The listing builds one solid part. Answer for the finished solid, in the listing's coordinates (mm). A direction names the side the tool comes from. Coordinates: 2 decimals unless noted, no trailing zeros. Order: outer loops, then holes, each group sorted by start corner. A loop starts at its lowest first (then second) coordinate and runs counter-clockwise, first axis right, second up. Notation, with made-up numbers: (49, 38.5) -> (94, 38.5) arc R17 cw to (94, 69.5) -> close; hole circle Ø1 at (75, -40). An arc over 180 degrees is marked (long way). Answer in a Markdown table with one row per item. Add a question column.
```python
from build123d import *

# Parameters (mm, degrees)
ESQUISSE1_W             = 200
ESQUISSE1_H             = 220
BOSS_EXTRU_1_DEPTH      = 15
ESQUISSE2_R             = 4
ENL_V_MAT_EXTRU_1_DEPTH = 6
ENL_V_MAT_EXTRU_2_DEPTH = 1.6
ENL_V_MAT_EXTRU_3_DEPTH = 5


with BuildPart() as part:
    # Esquisse1 → Boss.-Extru.1 (new body)
    with BuildSketch(Plane.XY):
        with Locations((100, 110)):
            Rectangle(ESQUISSE1_W, ESQUISSE1_H)
    extrude(amount=BOSS_EXTRU_1_DEPTH)

    # Esquisse2 → Enlèv. mat.-Extru.1 (cut)
    with BuildSketch(Plane.XY.offset(15)):
        with Locations((74.322, 91.45)):
            Circle(ESQUISSE2_R)
        with Locations((74.322, 153.45)):
            Circle(ESQUISSE2_R)
        with Locations((114.822, 91.45)):
            Circle(ESQUISSE2_R)
        with Locations((114.822, 153.45)):
            Circle(ESQUISSE2_R)
    extrude(amount=-ENL_V_MAT_EXTRU_1_DEPTH, mode=Mode.SUBTRACT)

    # Esquisse3 → Enlèv. mat.-Extru.2 (cut)
    with BuildSketch(Plane.XY.offset(15)):
        Polygon((27, 50), (27, 24.928776057), (74, 24.928776057), (74, 49.915697098), (124.85, 49.915697098), (124.85, 189.875697098), (25, 189.875697098), (25, 50), align=None)
    extrude(amount=-ENL_V_MAT_EXTRU_2_DEPTH, mode=Mode.SUBTRACT)

    # Esquisse4 → Enlèv. mat.-Extru.3 (cut)
    with BuildSketch(Plane.XY.offset(15)):
        with BuildLine():
            Line((106.85, 182.875697098), (101.85, 182.875697098))
            ThreePointArc((101.85, 182.875697098), (98.314466094, 181.411231003), (96.85, 177.875697098))
            Line((96.85, 177.875697098), (96.85, 65.875697098))
            ThreePointArc((96.85, 65.875697098), (98.314466094, 62.340163192), (101.85, 60.875697098))
            Line((101.85, 60.875697098), (106.85, 60.875697098))
            ThreePointArc((106.85, 60.875697098), (110.385533906, 62.340163192), (111.85, 65.875697098))
            Line((111.85, 65.875697098), (111.85, 177.875697098))
            ThreePointArc((111.85, 177.875697098), (110.385533906, 181.411231003), (106.85, 182.875697098))
        make_face()
        with BuildLine():
            Line((87.85, 60.875697098), (82.85, 60.875697098))
            ThreePointArc((82.85, 60.875697098), (79.314466094, 62.340163192), (77.85, 65.875697098))
            Line((77.85, 65.875697098), (77.85, 177.875697098))
            ThreePointArc((77.85, 177.875697098), (79.314466094, 181.411231003), (82.85, 182.875697098))
            Line((82.85, 182.875697098), (87.85, 182.875697098))
            ThreePointArc((87.85, 182.875697098), (91.385533906, 181.411231003), (92.85, 177.875697098))
            Line((92.85, 177.875697098), (92.85, 65.875697098))
            ThreePointArc((92.85, 65.875697098), (91.385533906, 62.340163192), (87.85, 60.875697098))
        make_face()
        with BuildLine():
            Line((65.85, 187.875697098), (58.85, 187.875697098))
            ThreePointArc((58.85, 187.875697098), (55.314466094, 186.411231003), (53.85, 182.875697098))
            Line((53.85, 182.875697098), (53.85, 77.875697098))
            ThreePointArc((53.85, 77.875697098), (55.314466094, 74.340163192), (58.85, 72.875697098))
            Line((58.85, 72.875697098), (65.85, 72.875697098))
            ThreePointArc((65.85, 72.875697098), (69.385533906, 74.340163192), (70.85, 77.875697098))
            Line((70.85, 77.875697098), (70.85, 182.875697098))
            ThreePointArc((70.85, 182.875697098), (69.385533906, 186.411231003), (65.85, 187.875697098))
        make_face()
    extrude(amount=-ENL_V_MAT_EXTRU_3_DEPTH, mode=Mode.SUBTRACT)


solid = part.part
```
Q1. Given pin 1 (4 mm diameter, centred on x = 75.5, y = 152.5, fed in from +Z); pin 2 (9 mm diameter, centred on x = 113.5, y = 90, fed in from +Z); pin 3 (5 mm diameter, centred on x = 60.5, y = 142.5, fed in from +Z), each flat-ended and moving along its own axis, determine where each tip first touches the part or whether it passes through.
Q2. A cutting plane is placed at A-A (y = 139). Determine the outline of the cut face in (x, z), then the cut area to 3 significant figures.
Q3. Determine the mould class of faces 3 (the face through (99, 0, 7)), 4 (the face through (99, 112, 0)), 5 (the face through (91.424, 62.379, 11.724)) for opening direction Y: +Y half, -Y half, draft (parallel to the pull), parting line (faces both ways), or undercut.
Q4. For faces 1 (the face through (143, 112, 15)), 2 (the face through (71.148, 151.016, 11.231)), determine the directions among +Z, -Z, +X, -X, +Y, -Y from which every point of the face is accessible in a straight line to the end or side of a thin tool.
Q5. Straight lines are drawn through the part: line 1 (X direction, y = 153.45, z = 11.05); line 2 (X direction, y = 163, z = 12.75); line 3 (X direction, y = 84, z = 14). For each, find the intervals that lie inside material, in ascending order.
Returned:
| question | item | result |
|---|---|---|
| 1 | pin 1 | stops at z = 9 |
| 1 | pin 2 | stops at z = 13.4 |
| 1 | pin 3 | stops at z = 10 |
| 2 | outline | (0, 0) -> (200, 0) -> (200, 15) -> (124.85, 15) -> (124.85, 13.4) -> (111.85, 13.4) -> (111.85, 10) -> (96.85, 10) -> (96.85, 13.4) -> (92.85, 13.4) -> (92.85, 10) -> (77.85, 10) -> (77.85, 13.4) -> (70.85, 13.4) -> (70.85, 10) -> (53.85, 10) -> (53.85, 13.4) -> (25, 13.4) -> (25, 15) -> (0, 15) -> close |
| 2 | area | 2,680 mm² |
| 3 | face 3 | -Y half |
| 3 | face 4 | draft |
| 3 | face 5 | undercut |
| 4 | face 1 | +Z, +X, -X, +Y, -Y |
| 4 | face 2 | +Z |
| 5 | line 1 | x = 0 to 53.85, 92.85 to 96.85, 118.82 to 200 |
| 5 | line 2 | x = 0 to 53.85, 70.85 to 77.85, 92.85 to 96.85, 111.85 to 200 |
| 5 | line 3 | x = 0 to 25, 124.85 to 200 |
